from build123d import *


with BuildPart() as part:
    # Sketch1 → Revolve2 (revolve)
    with BuildSketch(Plane.XY, mode=Mode.PRIVATE) as revolve2_sk:
        Polygon((-1.231630681, 0), (-5.431630681, 0), (-5.431630681, 33.4), (-3.138866015, 33.4), (-1.995791511, 32.7), (-3.138866015, 32.014155298), (-3.138866015, 30.22), (-1.995791511, 29.52), (-3.138866015, 28.834155298), (-3.138866015, 27.04), (-1.995791511, 26.34), (-3.138866015, 25.654155298), (-3.138866015, 23.86), (-1.995791511, 23.16), (-3.138866015, 22.474155298), (-3.138866015, 20.68), (-1.995791511, 19.98), (-3.138866015, 19.294155298), (-3.138866015, 17.5), (-1.995791511, 16.8), (-3.138866015, 16.114155298), (-3.138866015, 14.32), (-1.995791511, 13.62), (-3.138866015, 12.934155298), (-3.138866015, 11.14), (-1.995791511, 10.44), (-3.138866015, 9.754155298), (-3.138866015, 7.96), (-1.995791511, 7.26), (-1.231630681, 6.795995819), align=None)
    revolve(revolve2_sk.sketch.rotate(Axis((-5.431630681, 34.2, 0), (0, -1, 0)), 180), axis=Axis((-5.431630681, 34.2, 0), (0, -1, 0)))


solid = part.part
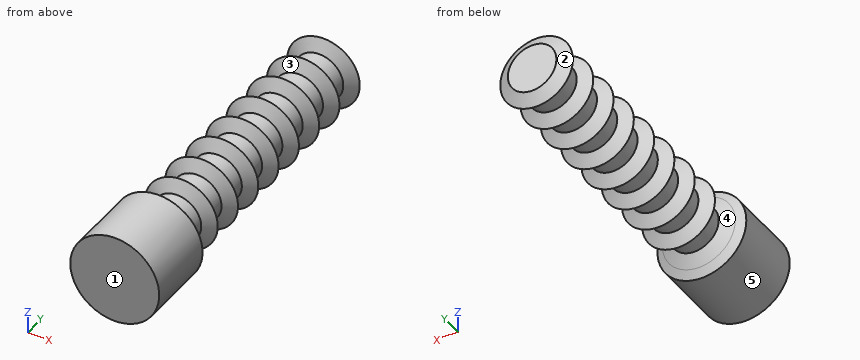
Can you work these out from the model? Positions are in its coordinate system, mm. Face numbers are marked on the shaded views. A direction names the side the tool comes from. Round coordinates to 2 decimals unless told otherwise and drop trailing zeros. Loops run counter-clockwise (first coordinate to the right, second up) from the corner with the lowest first, then second, coordinate; pieces in that order, holes last. Notation, with made-up numbers: (-16.75, 87) - (-5.75, 87) arc R9 ccw to (-5.75, 99) - close; hole circle Ø10 at (76.25, -18). An arc over 180 degrees is marked (long way). Use CSV: the item, a comma, the result in double quotes. Start each with the question number.
1) For the marked faces 4 and 5, which set-ups out of +Z, -Z, +X, -X, +Y, -Y let a thin tool reach every point of the face, with its end or its side?
2) If we section it at B-B on x = -2.5: Count the separate pieces of the cut face and the enclosed holes in it, plus the area to 3 significant figures.
3) If we section it at A-A on y = 15.5: Write out the boundary of the cut face in (x, z), plus the area to 3 significant figures.
4) Please list where these lines run through material, in increasing order: probe 1 along Z at (x, y) = (-5.25, 28); probe 2 along X at (y, z) = (11.5, -1.25); probe 3 along X at (y, z) = (17, -2). Write a range as [from, to].
5) We'd pull the mould along Y, two halves only. Please class the marked faces 1, 2 and 3: released by +Y, released by -Y, zero draft, split by the parting line, or undercut.
6) For pin 1 Ø5 at (y, z) = (19, 0.5) entering from +X; pin 2 Ø4 at (x, y) = (-6.5, 9.5) entering from +Z, each with a flat end and sliding along its axis, tell me the tip position at first contact or that it passes through.
Geometry results:
1,face 4,"none"
1,face 5,"+Y, -Y"
2,separate pieces,"9"
2,enclosed holes,"0"
2,area,"55.4 mm2"
3,outline,"circle Ø4.59 at (-5.43, 0)"
3,area,"16.5 mm2"
4,probe 1,"z = [-2.29, 2.29]"
4,probe 2,"x = [-7.35, -3.51]"
4,probe 3,"x = [-7.81, -3.05]"
5,face 1,"released by -Y"
5,face 2,"released by +Y"
5,face 3,"undercut"
6,pin 1,"stops at x = -2"
6,pin 2,"stops at z = 3.44"
